Work out the finished part from the listing and answer in its coordinate system (mm). A direction names the side the tool comes from. Round coordinates to 2 decimals unless told otherwise and drop trailing zeros. Loops run counter-clockwise (first coordinate to the right, second up) from the corner with the lowest first, then second, coordinate; pieces in that order, holes last. Notation, with made-up numbers: (56.25, 78.25) - (71.25, 78.25) arc R24 ccw to (71.25, 109.25) - close; hole circle Ø3 at (78.25, 63.25). An arc over 180 degrees is marked (long way). Return JSON: item names as keys, results as strings.
Autodesk Inventor part; units mm, degrees
ref_plane "YZ Plane" through (0, 0, 0) normal (1, 0, 0) x (0, 1, 0)
ref_plane "XZ Plane" through (0, 0, 0) normal (0, 1, 0) x (-1, 0, 0)
ref_plane "XY Plane" through (0, 0, 0) normal (0, 0, 1) x (1, 0, 0)
sketch "Sketch1" plane through (0, 0, 0) normal (0, 0, 1) x (1, 0, 0)
  circle A0 centre (0, 0) radius 24
  circle A1 centre (0, 0) radius 3.5
  arc A2 (7.6927, 7.8627) -> (-5.6038, 9.4656) centre (0, 0) ccw
  line L0 (0, 0) -> (7.6927, 7.8627) construction
  line L1 (0, 0) -> (-5.6038, 9.4656) construction
  arc A3 (13.2874, 13.5811) -> (-9.6793, 16.3497) centre (0, 0) ccw
  line L2 (0, 0) -> (13.2874, 13.5811) construction
  line L3 (0, 0) -> (-9.6793, 16.3497) construction
  line L4 (-5.6038, 9.4656) -> (-9.6793, 16.3497)
  line L5 (7.6927, 7.8627) -> (13.2874, 13.5811)
  arc A4 (5.1178, -18.2977) -> (18.9989, 0.2077) centre (0, 0) ccw
  line L6 (0, 0) -> (18.9989, 0.2077) construction
  line L7 (10.9993, 0.1202) -> (18.9989, 0.2077)
  line L8 (0, 0) -> (5.1178, -18.2977) construction
  line L9 (2.963, -10.5934) -> (5.1178, -18.2977)
  arc A5 (2.963, -10.5934) -> (10.9993, 0.1202) centre (0, 0) ccw
  arc A6 (-18.4052, 4.7167) -> (-9.3196, -16.5573) centre (0, 0) ccw
  line L10 (0, 0) -> (-9.3196, -16.5573) construction
  line L11 (-5.3956, -9.5858) -> (-9.3196, -16.5573)
  line L12 (0, 0) -> (-18.4052, 4.7167) construction
  line L13 (-10.6557, 2.7307) -> (-18.4052, 4.7167)
  arc A7 (-10.6557, 2.7307) -> (-5.3956, -9.5858) centre (0, 0) ccw
  circle A8 centre (-6.3997, 4.8004) radius 1
  line L14 (-6.3997, 4.8004) -> (0, 0) construction
  circle A9 centre (-0.9575, -7.9425) radius 1
  circle A10 centre (7.3571, 3.1421) radius 1
  dimension "d0" = 48
  dimension "d1" = 7
  dimension "d2" = 11
  dimension "a1" = 75
  dimension "d4" = 19
  dimension "d5" = 75
  dimension "d8" = 360
  dimension "d10" = 2
  dimension "d11" = 8
  dimension "d12" = 22.5
  dimension "d15" = 360
extrude "Extrusion1" add sketch "Sketch1" along normal blind 2
extrude "Extrusion2" add sketch "Sketch1" along normal blind 21 contours A1
sketch "Sketch2" plane through (0, 0, 21) normal (0, 0, 1) x (1, 0, 0)
  line L0 (-18.4052, 4.7167) -> (-10.6557, 2.7307)
  arc A0 (-10.6557, 2.7307) -> (-5.3956, -9.5858) centre (0, 0) ccw
  line L1 (-5.3956, -9.5858) -> (-9.3196, -16.5573)
  arc A1 (-18.4052, 4.7167) -> (-9.3196, -16.5573) centre (0, 0) ccw
  line L2 (5.1178, -18.2977) -> (2.963, -10.5934)
  arc A2 (2.963, -10.5934) -> (10.9993, 0.1202) centre (0, 0) ccw
  line L3 (10.9993, 0.1202) -> (18.9989, 0.2077)
  arc A3 (5.1178, -18.2977) -> (18.9989, 0.2077) centre (0, 0) ccw
  line L4 (-5.6038, 9.4656) -> (-9.6793, 16.3497)
  arc A4 (13.2874, 13.5811) -> (-9.6793, 16.3497) centre (0, 0) ccw
  line L5 (13.2874, 13.5811) -> (7.6927, 7.8627)
  arc A5 (7.6927, 7.8627) -> (-5.6038, 9.4656) centre (0, 0) ccw
  circle A6 centre (0, 0) radius 3.5
  circle A7 centre (7.3571, 3.1421) radius 1
  circle A8 centre (-0.9575, -7.9425) radius 1
  circle A9 centre (-6.3997, 4.8004) radius 1
  circle A10 centre (0, 0) radius 24
extrude "Extrusion3" add sketch "Sketch2" against normal blind 2
sketch "Sketch3" plane through (0, 0, 19) normal (0, 0, -1) x (-1, 0, 0)
  circle A0 centre (0, 0) radius 24
  circle A1 centre (-7.3571, 3.1421) radius 1
  circle A2 centre (0.9575, -7.9425) radius 1
  circle A3 centre (6.3997, 4.8004) radius 1
  arc A4 (9.3196, -16.5573) -> (18.4052, 4.7167) centre (0, 0) ccw
  line L0 (18.4052, 4.7167) -> (10.6557, 2.7307)
  arc A5 (5.3956, -9.5858) -> (10.6557, 2.7307) centre (0, 0) ccw
  line L1 (5.3956, -9.5858) -> (9.3196, -16.5573)
  arc A6 (-18.9989, 0.2077) -> (-5.1178, -18.2977) centre (0, 0) ccw
  line L2 (-5.1178, -18.2977) -> (-2.963, -10.5934)
  arc A7 (-10.9993, 0.1202) -> (-2.963, -10.5934) centre (0, 0) ccw
  line L3 (-10.9993, 0.1202) -> (-18.9989, 0.2077)
  arc A8 (5.6038, 9.4656) -> (-7.6927, 7.8627) centre (0, 0) ccw
  line L4 (5.6038, 9.4656) -> (9.6793, 16.3497)
  arc A9 (9.6793, 16.3497) -> (-13.2874, 13.5811) centre (0, 0) ccw
  line L5 (-13.2874, 13.5811) -> (-7.6927, 7.8627)
  circle A10 centre (0.9575, -7.9425) radius 1
  line L6 (-0.6354, -7.2622) -> (0.7502, -6.2229)
  line L7 (0.7502, -6.2229) -> (2.343, -6.9032)
  line L8 (2.343, -6.9032) -> (2.5503, -8.6228)
  line L9 (2.5503, -8.6228) -> (1.1648, -9.6621)
  line L10 (1.1648, -9.6621) -> (-0.4281, -8.9818)
  line L11 (-0.4281, -8.9818) -> (-0.6354, -7.2622)
  line L12 (0, 0) -> (0.9575, -7.9425) construction
  line L13 (0, 0) -> (6.3997, 4.8004) construction
  line L14 (7.9925, 4.1202) -> (6.607, 3.0808)
  line L15 (6.607, 3.0808) -> (5.0141, 3.7611)
  line L16 (5.0141, 3.7611) -> (4.8068, 5.4807)
  line L17 (7.7852, 5.8398) -> (7.9925, 4.1202)
  line L18 (4.8068, 5.4807) -> (6.1924, 6.52)
  line L19 (6.1924, 6.52) -> (7.7852, 5.8398)
  line L20 (0, 0) -> (-7.3571, 3.1421) construction
  line L21 (-7.5644, 4.8617) -> (-5.9716, 4.1814)
  line L22 (-5.9716, 4.1814) -> (-5.7643, 2.4618)
  line L23 (-5.7643, 2.4618) -> (-7.1498, 1.4225)
  line L24 (-8.95, 3.8223) -> (-7.5644, 4.8617)
  line L25 (-7.1498, 1.4225) -> (-8.7427, 2.1027)
  line L26 (-8.7427, 2.1027) -> (-8.95, 3.8223)
  dimension "d23" = 3
  dimension "d26" = 360
extrude "Extrusion4" add sketch "Sketch3" along normal blind 17 contours L6 L7 L8 L9 L10 L11 | L14 L15 L16 L18 L19 L17 | L21 L22 L23 L25 L26 L24
sketch "Sketch4" plane through (0, 0, 21) normal (0, 0, 1) x (1, 0, 0)
  circle A0 centre (0, 0) radius 3.25
  dimension "d30" = 6.5
extrude "Extrusion5" add sketch "Sketch4" along normal blind 18.5
equation "\"d5\" = a1"
properties part number "platform_wheel"
1) Section A-A (x = -17) is taken. Give the vertices of the cut face in (y, z).
Verdict:
{"outline": "(-16.94, 0) - (-8.49, 0) - (-8.49, 2) - (-16.94, 2) - close; (-16.94, 19) - (-8.49, 19) - (-8.49, 21) - (-16.94, 21) - close; (4.36, 0) - (16.94, 0) - (16.94, 2) - (4.36, 2) - close; (4.36, 19) - (16.94, 19) - (16.94, 21) - (4.36, 21) - close"}
2) Section B-B (z = 15) is taken. Give the vertices of the cut face in (x, y).
Verdict:
{"outline": "(-7.99, 4.12) - (-6.61, 3.08) - (-5.01, 3.76) - (-4.81, 5.48) - (-6.19, 6.52) - (-7.79, 5.84) - close; circle Ø7 at (0, 0); (-2.55, -8.62) - (-1.16, -9.66) - (0.43, -8.98) - (0.64, -7.26) - (-0.75, -6.22) - (-2.34, -6.9) - close; (5.76, 2.46) - (7.15, 1.42) - (8.74, 2.1) - (8.95, 3.82) - (7.56, 4.86) - (5.97, 4.18) - close; hole circle Ø2 at (-6.4, 4.8); hole circle Ø2 at (-0.96, -7.94); hole circle Ø2 at (7.36, 3.14)"}
3) A tool of negligible diameter and unlimited length cuts with its end or side. For faces 1 (the flat face through (-7.613, 12.859, 0.986)), 2 (the flat face through (-5.5, 6, 10.6)), 3 (the flat face through (6.447, 1.949, 10.619)), from which of +Z, -Z, +X, -X, +Y, -Y can it reach the whole face along a straight path? Write none if from no direction.
Verdict:
{"face 1": "+Z, -Z", "face 2": "+X, +Y", "face 3": "-Y"}
4) Section D-D (x = 12.5) is taken. Give the vertices of the cut face in (y, z).
Verdict:
{"outline": "(-20.49, 0) - (-14.31, 0) - (-14.31, 2) - (-20.49, 2) - close; (-20.49, 19) - (-14.31, 19) - (-14.31, 21) - (-20.49, 21) - close; (0.14, 0) - (12.78, 0) - (12.78, 2) - (0.14, 2) - close; (0.14, 19) - (12.78, 19) - (12.78, 21) - (0.14, 21) - close; (14.31, 0) - (20.49, 0) - (20.49, 2) - (14.31, 2) - close; (14.31, 19) - (20.49, 19) - (20.49, 21) - (14.31, 21) - close"}
5) Find the intervals of material crossed by L1, parallel to Z at x = 4, y = -9; L2, parallel to Y at x = 8, z = 7.5; L3, parallel to Y at x = -1, z = 22, in increasing order.
Verdict:
{"L1": "z = 0 to 2, 19 to 21", "L2": "y = 1.79 to 2.38, 3.91 to 4.53", "L3": "y = -3.09 to 3.09"}
6) Section C-C (y = -14) is taken. Give the vertices of the cut face in (x, z), and give its area (3 significant figures).
Verdict:
{"outline": "(-19.49, 0) - (-12.85, 0) - (-12.85, 2) - (-19.49, 2) - close; (-19.49, 19) - (-12.85, 19) - (-12.85, 21) - (-19.49, 21) - close; (-7.88, 0) - (3.92, 0) - (3.92, 2) - (-7.88, 2) - close; (-7.88, 19) - (3.92, 19) - (3.92, 21) - (-7.88, 21) - close; (12.85, 0) - (19.49, 0) - (19.49, 2) - (12.85, 2) - close; (12.85, 19) - (19.49, 19) - (19.49, 21) - (12.85, 21) - close", "area": "100 mm2"}
7) Determine the mould class of faces 4 (the flat face through (8.845, 2.95, 10.619)), 5 (the cylindrical face through (15.303, -11.261, 0.986)), 6 (the flat face through (-6.978, 6.185, 10.619)) for opening direction X: pulls with the +X half, pulls with the -X half, needs draft (parallel to the pull), parting line crosses it, or undercut.
Verdict:
{"face 4": "pulls with the +X half", "face 5": "undercut", "face 6": "pulls with the -X half"}
8) Flat-ended cylindrical pins translate along their axes: pin 1 (10 mm diameter, centred on x = 1.5, y = -11.5, fed in from -Z); pin 2 (12 mm diameter, centred on x = -7, y = -6.5, fed in from +Z); pin 3 (3 mm diameter, centred on x = 7.5, z = 7, fed in from +Y); pin 4 (12 mm diameter, centred on x = -4.5, z = 15.5, fed in from -Y). Find the tip coordinate at first contact, or state that the pin passes through.
Verdict:
{"pin 1": "stops at z = 0", "pin 2": "stops at z = 21", "pin 3": "stops at y = 4.86", "pin 4": "stops at y = -24"}
